Check sheet for the modelled part. Datum: model origin and axes. Units: mm. Give positions to 0.01 mm unless a question says otherwise; leave off trailing zeros. Loops run counter-clockwise (first coordinate to the right, second up) from the corner with the lowest first, then second, coordinate; pieces in that order, holes last. Notation, with made-up numbers: (10.25, 45.5) -> (29.25, 45.5) arc R17 ccw to (29.25, 70.5) -> close; hole circle Ø3 at (17, 62). An arc over 180 degrees is marked (long way). Write each question's results on one line, items separated by ' | '. Start each with the question number.
Item 1: Mould release check, pull along X, two halves, no side actions. Record for faces 1 (the face through (-8, 8, 0)), 2 (the face through (-10, 8, -0.5)), 3 (the face through (-20.75, 7.8, 0.5)): pulls with the +X half, pulls with the -X half, needs draft (parallel to the pull), parting line crosses it, or undercut.
Item 2: Cross-section at B-B on x = -16.65. Enter the section's corners in (y, z).
Item 3: Cross-section at A-A on z = 5. Enter the section's corners in (x, y), then the cut area to 3 significant figures.
Item 4: Gauge pin test, flat ends, axial feed: pin 1 Ø1.5 at (x, z) = (-3.5, 5) entering from +Y; pin 2 Ø0.6 at (x, z) = (-6.5, -0.5) entering from -Y (3 decimals); pin 3 Ø4 at (x, y) = (-2.5, 12) entering from +Z; pin 4 Ø3 at (y, z) = (12, 3) entering from -X. Record the tip position at first contact, or that the pin passes through.
Item 5: Scan lines: line 1 along Y through (x, z) = (-1.75, 0.35); line 2 along Z through (x, y) = (-11.5, 9.75); line 3 along Z through (x, y) = (-2.75, 15.25). Record each from-to range of solid material in increasing order.
Item 6: Cross-section at D-D on z = 0.75. Enter the section's corners in (x, y), then the cut area to 3 significant figures.
Item 7: Cross-section at C-C on x = -2.25. Enter the section's corners in (y, z).
from build123d import *

# Parameters (mm, degrees)
ESQUISSE1_W             = 20.75
ESQUISSE1_H             = 15.75
BOSS_EXTRU_1_DEPTH      = 1
ESQUISSE4_W             = 0.5
ESQUISSE4_H             = 2
ESQUISSE4_H_2           = 1
ESQUISSE4_W_2           = 2.5
ESQUISSE4_W_3           = 4
ESQUISSE4_H_3           = 4
BOSS_EXTRU_4_DEPTH      = 0.5
ESQUISSE5_R             = 1.5
ENL_V_MAT_EXTRU_1_DEPTH = 5
ESQUISSE6_W             = 2.5
ESQUISSE6_H             = 2
BOSS_EXTRU_5_DEPTH      = 0.5
BOSS_EXTRU_6_DEPTH      = 5
BOSS_EXTRU_6_DEPTH_BACK = 1.5
ESQUISSE7_R             = 0.25


with BuildPart() as part:
    # Esquisse1 → Boss.-Extru.1 (new body)
    with BuildSketch(Plane.XY):
        with Locations((-10.375, 7.875)):
            Rectangle(ESQUISSE1_W, ESQUISSE1_H)
    extrude(amount=BOSS_EXTRU_1_DEPTH)

    # Esquisse4 → Boss.-Extru.4 (add)
    with BuildSketch(Plane(origin=(0, 0, 0), x_dir=(-1, 0, 0), z_dir=(0, 0, -1))):
        with Locations((6.625, 8.875)):
            Rectangle(ESQUISSE4_W, ESQUISSE4_H)
        with Locations((5.625, 9.375)):
            Rectangle(ESQUISSE4_W, ESQUISSE4_H_2)
        with Locations((4.625, 8.875)):
            Rectangle(ESQUISSE4_W, ESQUISSE4_H)
        with Locations((4.625, 6.375)):
            Rectangle(ESQUISSE4_W, ESQUISSE4_H_2)
        with Locations((6.625, 5.875)):
            Rectangle(ESQUISSE4_W, ESQUISSE4_H)
        with Locations((10.00670855, 3.574144423)):
            Rectangle(ESQUISSE4_W_2, ESQUISSE4_H_2)
        with Locations((10.375, 7.875)):
            Rectangle(ESQUISSE4_W_3, ESQUISSE4_H_3)
        with Locations((14.125, 8.875)):
            Rectangle(ESQUISSE4_W, ESQUISSE4_H)
        with Locations((16.125, 8.875)):
            Rectangle(ESQUISSE4_W, ESQUISSE4_H)
        with Locations((15.125, 9.375)):
            Rectangle(ESQUISSE4_W, ESQUISSE4_H_2)
        with Locations((14.125, 6.375)):
            Rectangle(ESQUISSE4_W, ESQUISSE4_H_2)
        with Locations((16.125, 5.875)):
            Rectangle(ESQUISSE4_W, ESQUISSE4_H)
    extrude(amount=BOSS_EXTRU_4_DEPTH)

    # Esquisse5 → Enlèv. mat.-Extru.1 (cut)
    with BuildSketch(Plane(origin=(0, 0, 0), x_dir=(-1, 0, 0), z_dir=(0, 0, -1))):
        with Locations((1.75, 1.75)):
            Circle(ESQUISSE5_R)
        with Locations((19, 1.75)):
            Circle(ESQUISSE5_R)
    extrude(amount=-ENL_V_MAT_EXTRU_1_DEPTH, mode=Mode.SUBTRACT)

    # Esquisse6 → Boss.-Extru.5 (add)
    with BuildSketch(Plane(origin=(0, 0, 0), x_dir=(-1, 0, 0), z_dir=(0, 0, -1))):
        with Locations((19, 8.875)):
            Rectangle(ESQUISSE6_W, ESQUISSE6_H)
    extrude(amount=BOSS_EXTRU_5_DEPTH)

    # Esquisse7 → Boss.-Extru.6 (add, two sides: drawn at the far end of the back side and taken through both)
    with BuildSketch(Plane.XY.offset(1).offset(-BOSS_EXTRU_6_DEPTH_BACK)):
        with Locations((-19.15, 14.5)):
            Circle(ESQUISSE7_R)
        with Locations((-16.65, 14.5)):
            Circle(ESQUISSE7_R)
        with Locations((-14.15, 14.5)):
            Circle(ESQUISSE7_R)
        with Locations((-11.65, 14.5)):
            Circle(ESQUISSE7_R)
        with Locations((-9.15, 14.5)):
            Circle(ESQUISSE7_R)
        with Locations((-6.65, 14.5)):
            Circle(ESQUISSE7_R)
        with Locations((-4.15, 14.5)):
            Circle(ESQUISSE7_R)
        with Locations((-1.65, 14.5)):
            Circle(ESQUISSE7_R)
    extrude(amount=BOSS_EXTRU_6_DEPTH + BOSS_EXTRU_6_DEPTH_BACK)


solid = part.part
Answer sheet:
1) face 1: undercut | face 2: needs draft | face 3: pulls with the -X half
2) outline: (0, 0) -> (14.25, 0) -> (14.25, -0.5) -> (14.75, -0.5) -> (14.75, 0) -> (15.75, 0) -> (15.75, 1) -> (14.75, 1) -> (14.75, 6) -> (14.25, 6) -> (14.25, 1) -> (0, 1) -> close
3) outline: circle Ø0.5 at (-19.15, 14.5); circle Ø0.5 at (-16.65, 14.5); circle Ø0.5 at (-14.15, 14.5); circle Ø0.5 at (-11.65, 14.5); circle Ø0.5 at (-9.15, 14.5); circle Ø0.5 at (-6.65, 14.5); circle Ø0.5 at (-4.15, 14.5); circle Ø0.5 at (-1.65, 14.5) | area: 1.57 mm²
4) pin 1: stops at y = 14.75 | pin 2: stops at y = 4.875 | pin 3: stops at z = 1 | pin 4: passes through
5) line 1: y = 0 to 0.25, 3.25 to 15.75 | line 2: z = -0.5 to 1 | line 3: z = 0 to 1
6) outline: (-20.75, 0) -> (0, 0) -> (0, 15.75) -> (-20.75, 15.75) -> close; hole circle Ø3 at (-19, 1.75); hole circle Ø3 at (-1.75, 1.75) | area: 313 mm²
7) outline: (0, 0) -> (0.34, 0) -> (0.34, 1) -> (0, 1) -> close; (3.16, 0) -> (15.75, 0) -> (15.75, 1) -> (3.16, 1) -> close
